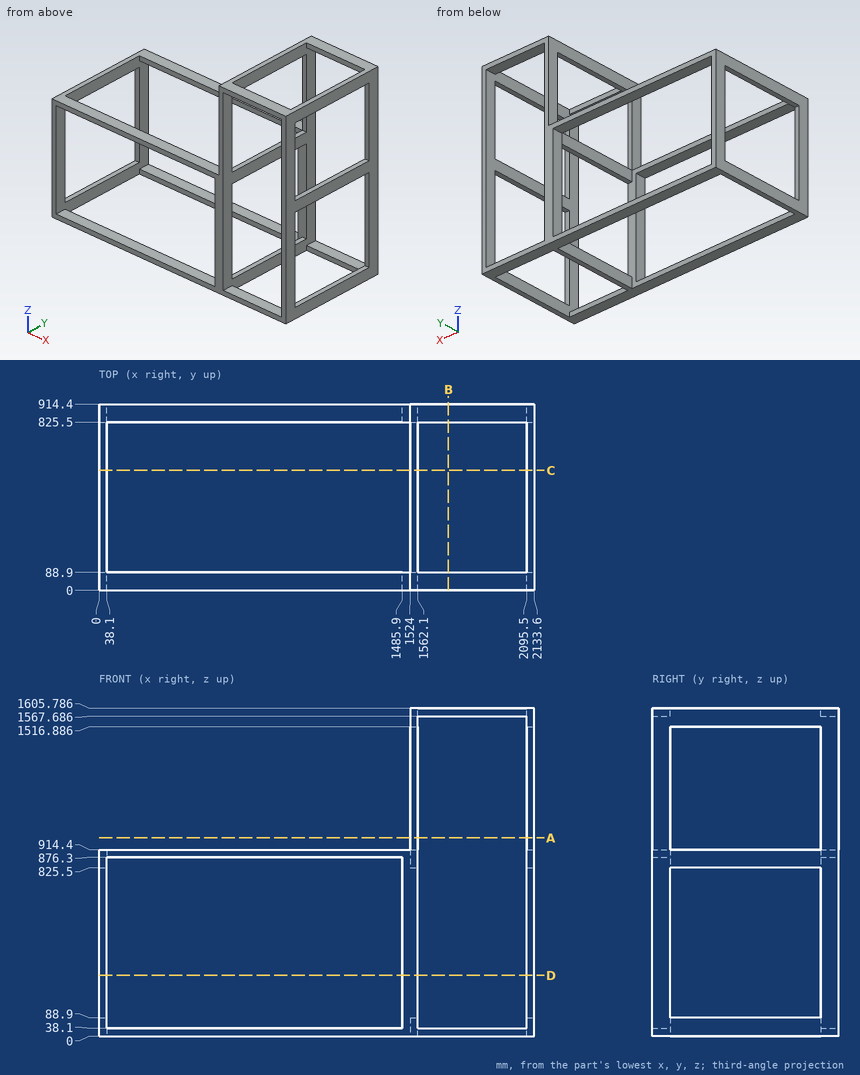
The figure shows three views and two pictorial views of one solid part (mm, origin at its lowest corner). Answer the questions. Coordinates: 2 decimals unless noted, no trailing zeros. Loops run counter-clockwise (first coordinate to the right, second up) from the corner with the lowest first, then second, coordinate; pieces in that order, holes last. Notation, with made-up numbers: (-38.75, 14) - (15.25, 14) arc R32 cw to (15.25, 52) - close; hole circle Ø11 at (16.25, 46). An arc over 180 degrees is marked (long way). Answer in a Markdown table with one row per item.
Q1. Find section B-B on x = 1712.5. Write down the section's boundary in (y, z).
Here are the results:
| item | result |
|---|---|
| outline | (0, 0) - (88.9, 0) - (88.9, 38.1) - (0, 38.1) - close; (0, 1567.69) - (88.9, 1567.69) - (88.9, 1605.79) - (0, 1605.79) - close; (825.5, 0) - (914.4, 0) - (914.4, 38.1) - (825.5, 38.1) - close; (825.5, 1567.69) - (914.4, 1567.69) - (914.4, 1605.79) - (825.5, 1605.79) - close |
Q2. Find section A-A on z = 972. Write down the section's boundary in (x, y).
Here are the results:
| item | result |
|---|---|
| outline | (1524, 0) - (1562.1, 0) - (1562.1, 88.9) - (1524, 88.9) - close; (1524, 825.5) - (1562.1, 825.5) - (1562.1, 914.4) - (1524, 914.4) - close; (2095.5, 0) - (2133.6, 0) - (2133.6, 88.9) - (2095.5, 88.9) - close; (2095.5, 825.5) - (2133.6, 825.5) - (2133.6, 914.4) - (2095.5, 914.4) - close |
Q3. Find section D-D on z = 297.5. Write down the section's boundary in (x, y), plus the area to 3 significant figures.
Here are the results:
| item | result |
|---|---|
| outline | (0, 0) - (38.1, 0) - (38.1, 88.9) - (0, 88.9) - close; (0, 825.5) - (38.1, 825.5) - (38.1, 914.4) - (0, 914.4) - close; (1485.9, 0) - (1562.1, 0) - (1562.1, 88.9) - (1485.9, 88.9) - close; (1485.9, 825.5) - (1562.1, 825.5) - (1562.1, 914.4) - (1485.9, 914.4) - close; (2095.5, 0) - (2133.6, 0) - (2133.6, 88.9) - (2095.5, 88.9) - close; (2095.5, 825.5) - (2133.6, 825.5) - (2133.6, 914.4) - (2095.5, 914.4) - close |
| area | 27,100 mm^2 |
Q4. Straight lines are drawn through the part: line 1 along X through (y, z) = (829, 328.5); line 2 along Y through (x, z) = (1533.5, 284); line 3 along Z through (x, y) = (1548, 479). For each, find the intervals that lie inside material, in ascending order. Write a range as [from, to].
Here are the results:
| item | result |
|---|---|
| line 1 | x = [0, 38.1], [1485.9, 1562.1], [2095.5, 2133.6] |
| line 2 | y = [0, 88.9], [825.5, 914.4] |
| line 3 | z = [0, 88.9], [825.5, 914.4], [1516.89, 1605.79] |
Q5. Given P1, Ø19, axis at x = 22.5, y = 430.5, coming from the +Z side, flat-ended and moving along its own axis, determine where the tip first touches the part or whether it passes through.
Here are the results:
| item | result |
|---|---|
| P1 | stops at z = 914.4 |
Q6. Find section C-C on y = 588.5. Count the separate pieces of the cut face and the enclosed holes in it, plus the area to 3 significant figures.
Here are the results:
| item | result |
|---|---|
| separate pieces | 8 |
| enclosed holes | 0 |
| area | 27,100 mm^2 |
